The figure shows three views and two pictorial views of one solid part (mm, origin at its lowest corner). Answer the questions. A direction names the side the tool comes from. Round coordinates to 2 decimals unless told otherwise and drop trailing zeros. Order: outer loops, then holes, each group sorted by start corner. A loop starts at its lowest first (then second) coordinate and runs counter-clockwise, first axis right, second up. Notation, with made-up numbers: (70.5, 51.25) - (115.5, 51.25) arc R20 cw to (115.5, 87.25) - close; hole circle Ø10 at (59.5, 70.5). An arc over 180 degrees is marked (long way). One line per item, written item: value. Start each with the question number.
1. A tool of negligible diameter and unlimited length cuts with its end or side. For the marked faces 1, 2, 3 and 4, from which of +Z, -Z, +X, -X, +Y, -Y can it reach the whole face along a straight path? Write none if from no direction.
2. Flat-ended cylindrical pins translate along their axes: P1, Ø2, axis at x = 10, y = 5, coming from the +Z side; P2, Ø3, axis at y = 5, z = 10, coming from the +X side. Find the tip coordinate at first contact, or state that the pin passes through.
3. Straight lines are drawn through the part: line 1 (Y direction, x = 10, z = 16.25); line 2 (Z direction, x = 3.75, y = 5). For each, find the intervals that lie inside material, in ascending order.
4. Section A-A, the plane x = 1.5 is taken. Give the vertices of the cut face in (y, z) (1 decimal), then the cut area to 3 significant figures.
5. For a pull along Z with two mould halves and no side action, classify the marked faces 5, 6, 7 and 8 as released by +Z, released by -Z, zero draft, split by the parting line, or undercut.
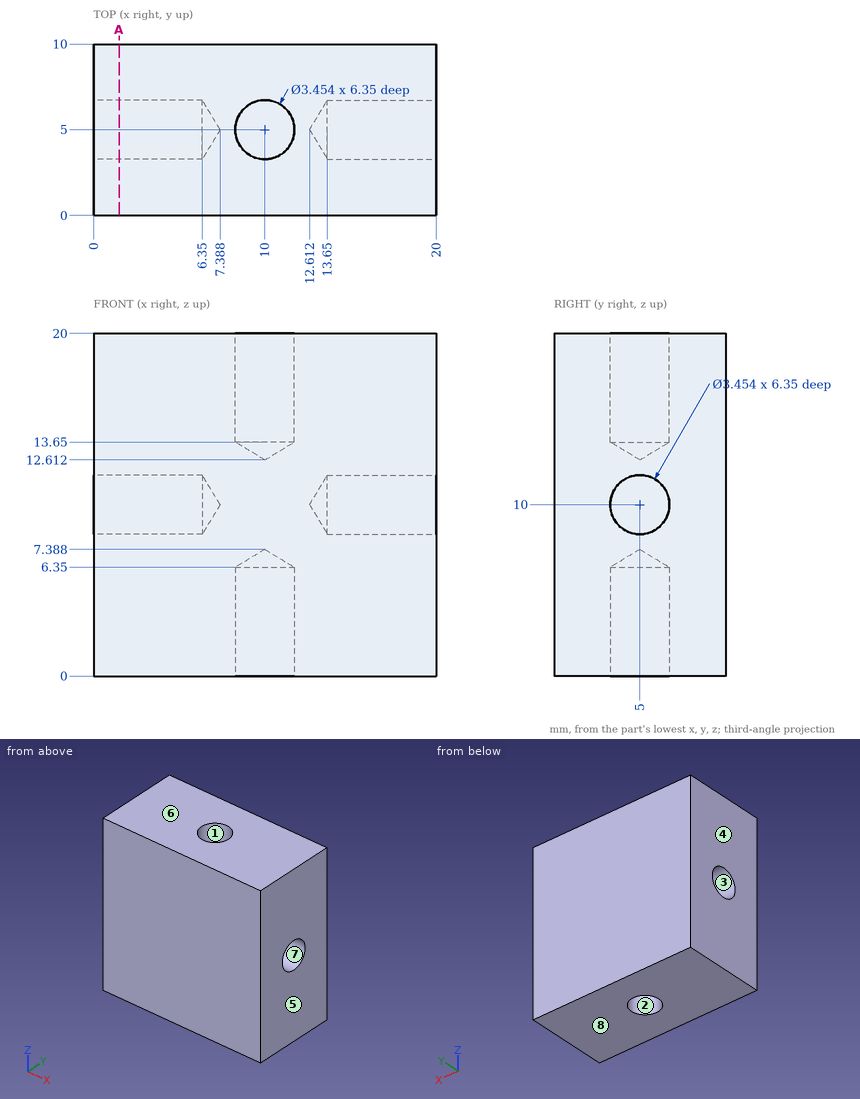
Answer list:
1. face 1: +Z
1. face 2: -Z
1. face 3: -X
1. face 4: +Z, -Z, -X, +Y, -Y
2. P1: stops at z = 13.21
2. P2: stops at x = 13.51
3. line 1: y = 0 to 3.27, 6.73 to 10
3. line 2: z = 0 to 8.27, 11.73 to 20
4. outline: (0, 0) - (10, 0) - (10, 20) - (0, 20) - close; hole circle Ø3.5 at (5, 10)
4. area: 191 mm²
5. face 5: zero draft
5. face 6: released by +Z
5. face 7: undercut
5. face 8: released by -Z
